Verification items for the finished model (mm, model axes). Face numbers are marked on the shaded views. A direction names the side the tool comes from. Coordinates: 2 decimals unless noted, no trailing zeros. Order: outer loops, then holes, each group sorted by start corner. A loop starts at its lowest first (then second) coordinate and runs counter-clockwise, first axis right, second up. Notation, with made-up numbers: (12.25, 25) -> (49.25, 25) arc R21 cw to (49.25, 29) -> close; hole circle Ø5 at (66, 82.5). An arc over 180 degrees is marked (long way). Write each question's results on one line, items separated by ' | '. Start each with the question number.
(1) Set-up check for the marked faces 5, 6 and 7: record each of +Z, -Z, +X, -X, +Y, -Y from which the full face is reachable in a straight line by a thin tool's end or side.
(2) Cross-section at C-C on x = 21.5. Enter the section's corners in (y, z), and give its area (3 significant figures).
(3) Thickness scan on probe 1 along X at (y, z) = (47, 6); probe 2 along X at (y, z) = (50.5, 0.5); probe 3 along X at (y, z) = (61, 1). Record the ranges inside material, lowest first. Write a range as [from, to].
(4) Cross-section at D-D on y = 63. Enter the section's corners in (x, z), and give its area (3 significant figures).
(5) Draft check along X on the marked faces 1, 2, 3 and 4. Enter one of: +X half, -X half, draft (parallel to the pull), parting line (faces both ways), or undercut.
(6) Cross-section at B-B on z = 6.5. Enter the section's corners in (x, y), and give its area (3 significant figures).
(7) Cross-section at A-A on x = 27.5. Enter the section's corners in (y, z), and give its area (3 significant figures).
(8) Go/stop test with flat-tipped pins: pin 1 (4 mm diameter, centred on y = 39, z = 2.5, fed in from +X); pin 2 (3 mm diameter, centred on x = 25.5, z = 3, fed in from -Y); pin 3 (1.5 mm diameter, centred on x = 22.5, z = 1, fed in from -Y). Record where each tip stops, or that it passes through.
```python
from build123d import *

# Parameters (mm, degrees)
PAD_DEPTH       = 8
POCKET_DEPTH    = 4
SKETCH002_R     = 1.5
SKETCH002_W     = 14
SKETCH002_H     = 5
SKETCH002_W_2   = 6
SKETCH002_H_2   = 6
POCKET001_DEPTH = 5


with BuildPart() as part:
    # Sketch → Pad (new body)
    with BuildSketch(Plane.XY):
        with BuildLine():
            Line((10, 80), (10, 80.00008))
            Line((10, 80.00008), (45, 80.00008))
            Line((45, 80.00008), (45, 45.00008))
            ThreePointArc((10, 45), (27.50004, 27.500049), (45, 45.00008))
            Line((10, 45), (10, 80))
        make_face()
    extrude(amount=PAD_DEPTH)

    # Sketch001 (on Face7 of Pad) → Pocket (cut)
    with BuildSketch(Plane.XY.offset(8)):
        with BuildLine():
            Line((12.5, 80.00008), (12.5, 45))
            ThreePointArc((12.5, 45), (27.50004, 30), (42.5, 45.00008))
            Line((42.5, 45.00008), (42.5, 80.00008))
            Line((42.5, 80.00008), (12.5, 80.00008))
        make_face()
    extrude(amount=-POCKET_DEPTH, mode=Mode.SUBTRACT)

    # Sketch002 (on Face9 of Pocket) → Pocket001 (cut)
    with BuildSketch(Plane.XY.offset(4)):
        with Locations((17.5, 60.00008)):
            Circle(SKETCH002_R)
        with Locations((37.5, 60.00008)):
            Circle(SKETCH002_R)
        with Locations((27, 49.50008)):
            Rectangle(SKETCH002_W, SKETCH002_H)
        with Locations((27.5, 70.00008)):
            Rectangle(SKETCH002_W_2, SKETCH002_H_2)
    extrude(amount=-POCKET001_DEPTH, mode=Mode.SUBTRACT)


solid = part.part
```
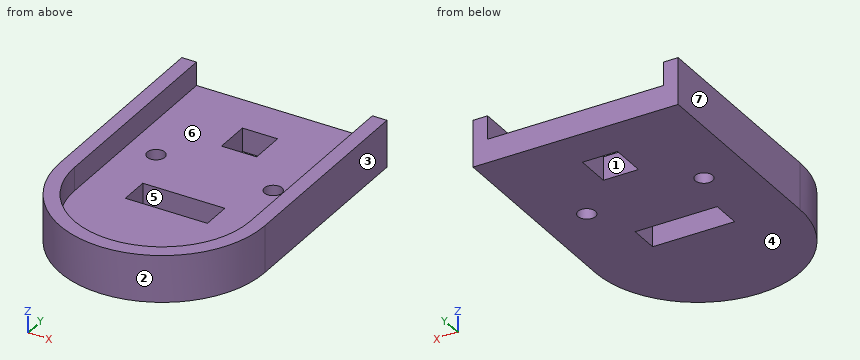
Results are:
1) face 5: +Z, -Z | face 6: +Z, +Y | face 7: +Z, -Z, -X, +Y, -Y
2) outline: (28.56, 0) -> (47, 0) -> (47, 4) -> (31.25, 4) -> (31.25, 8) -> (28.56, 8) -> close; (52, 0) -> (80, 0) -> (80, 4) -> (52, 4) -> close | area: 197 mm2
3) probe 1: x = [10, 12.5], [42.5, 45] | probe 2: x = [10, 20], [34, 45] | probe 3: x = [10, 16.38], [18.62, 36.38], [38.62, 45]
4) outline: (10, 0) -> (45, 0) -> (45, 8) -> (42.5, 8) -> (42.5, 4) -> (12.5, 4) -> (12.5, 8) -> (10, 8) -> close | area: 160 mm2
5) face 1: undercut | face 2: parting line | face 3: +X half | face 4: draft
6) outline: (10, 45) arc R17.5 ccw to (45, 45) -> (45, 80) -> (42.5, 80) -> (42.5, 45) arc R15 cw to (12.5, 45) -> (12.5, 80) -> (10, 80) -> close | area: 303 mm2
7) outline: (27.5, 0) -> (47, 0) -> (47, 4) -> (30, 4) -> (30, 8) -> (27.5, 8) -> close; (52, 0) -> (67, 0) -> (67, 4) -> (52, 4) -> close; (73, 0) -> (80, 0) -> (80, 4) -> (73, 4) -> close | area: 176 mm2
8) pin 1: stops at x = 44.54 | pin 2: stops at y = 27.51 | pin 3: stops at y = 28.02
